Check sheet for the drawn part. Datum: minimum x, y, z corner. Units: mm. A direction names the side the tool comes from. Round coordinates to 2 decimals unless told otherwise and drop trailing zeros. Write each loop counter-clockwise with the first axis right and the second up, starting at its lowest first coordinate (ties: lowest second). Pieces come first, ordered by that corner, then holes. Notation, with made-up numbers: (12.25, -11.5) -> (53.25, -11.5) arc R25 ccw to (53.25, 19.5) -> close; hole circle Ø2 at (-24.75, 9.5). An arc over 180 degrees is marked (long way). One line per item, written item: value. Start each with the question number.
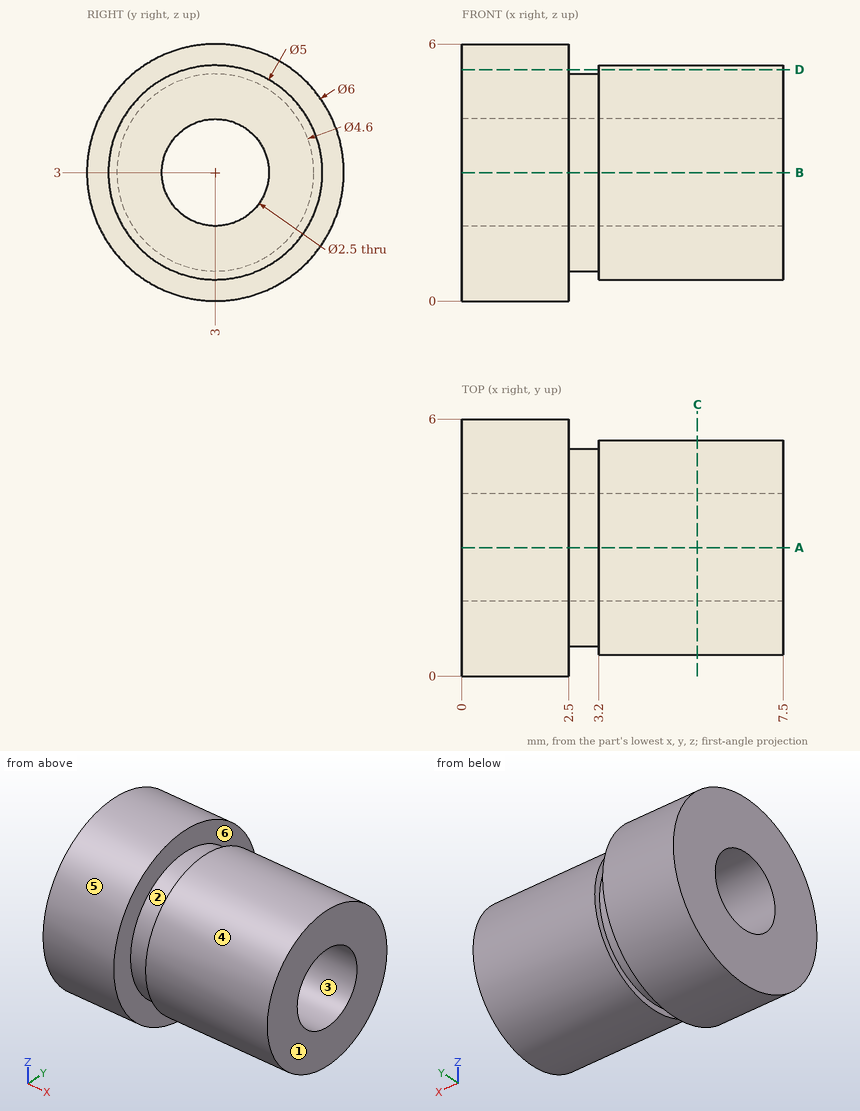
1. Depth check by flat-ended pin: pin 1 Ø1 at (x, y) = (1.5, 5.5) entering from -Z; pin 2 Ø1 at (x, y) = (4.5, 1) entering from -Z; pin 3 Ø1.5 at (y, z) = (3, 3) entering from -X; pin 4 Ø1 at (x, y) = (6.5, 1.5) entering from +Z. Enter the tip coordinate at first touch or a pass-through.
2. Material ranges on probe 1 along X at (y, z) = (3.75, 5.35); probe 2 along X at (y, z) = (5.55, 2.85); probe 3 along Y at (x, z) = (4.75, 3.7), recorded low to high.
3. Release check for a two-part mould opening along Y. For the marked faces 1, 2 and 3 record: +Y half, -Y half, draft (parallel to the pull), parting line (faces both ways), or undercut.
4. Cross-section at D-D (z = 5.4). Record the cut outline in (x, y), plus the area to 3 significant figures.
5. Access from +Z, -Z, +X, -X, +Y, -Y to the whole of each face (thin tool, end or side, straight path). Record for the marked faces 4, 5 and 6.
6. Cross-section at C-C (x = 5.5). Record the cut outline in (y, z), plus the area to 3 significant figures.
7. Cross-section at A-A (y = 3). Record the cut outline in (x, z).
Working result:
1. pin 1: stops at z = 0.76
1. pin 2: stops at z = 1
1. pin 3: passes through
1. pin 4: stops at z = 5.29
2. probe 1: x = 0 to 2.5, 3.2 to 7.5
2. probe 2: x = 0 to 2.5
2. probe 3: y = 0.6 to 1.96, 4.04 to 5.4
3. face 1: draft
3. face 2: parting line
3. face 3: undercut
4. outline: (0, 1.2) -> (2.5, 1.2) -> (2.5, 4.8) -> (0, 4.8) -> close; (3.2, 2.3) -> (7.5, 2.3) -> (7.5, 3.7) -> (3.2, 3.7) -> close
4. area: 15.0 mm^2
5. face 4: +X
5. face 5: +X, -X
5. face 6: none
6. outline: circle Ø5 at (3, 3); hole circle Ø2.5 at (3, 3)
6. area: 14.7 mm^2
7. outline: (0, 0) -> (2.5, 0) -> (2.5, 0.7) -> (3.2, 0.7) -> (3.2, 0.5) -> (7.5, 0.5) -> (7.5, 1.75) -> (0, 1.75) -> close; (0, 4.25) -> (7.5, 4.25) -> (7.5, 5.5) -> (3.2, 5.5) -> (3.2, 5.3) -> (2.5, 5.3) -> (2.5, 6) -> (0, 6) -> close
